```python
from build123d import *

# Parameters (mm, degrees)
CHAMFER_1_SIZE = 0.2
CHAMFER_2_SIZE = 0.1


with BuildPart() as part:
    # Эскиз1 → Повернуть1 (revolve)
    with BuildSketch(Plane.XY, mode=Mode.PRIVATE) as revolve_1_sk:
        Polygon((0, 0), (26, 0), (26, 2), (25, 2), (25, 1.7), (24.3, 1.7), (24.3, 2), (8, 2), (8, 3), (5.5, 3), (5.5, 2), (0, 2), align=None)
    revolve(revolve_1_sk.sketch.rotate(Axis((0, 0, 0), (1, 0, 0)), 90), axis=Axis((0, 0, 0), (1, 0, 0)))

    # Фаска1
    chamfer_1_edges = [part.edges().sort_by_distance(p)[0] for p in [
        (26, 0, -2),
        (0, 0, -2),
    ]]
    chamfer(chamfer_1_edges, length=CHAMFER_1_SIZE)

    # Фаска2
    chamfer_2_edges = [part.edges().sort_by_distance(p)[0] for p in [
        (24.3, 0, -2),
        (25, 0, -2),
    ]]
    chamfer(chamfer_2_edges, length=CHAMFER_2_SIZE)


solid = part.part
```
Geometry: final body of the model. Coordinates: model frame, mm. A direction names the side the tool comes from. Round coordinates to 2 decimals unless told otherwise and drop trailing zeros. Order: outer loops, then holes, each group sorted by start corner. A loop starts at its lowest first (then second) coordinate and runs counter-clockwise, first axis right, second up. Notation, with made-up numbers: (24, 8.5) -> (32, 8.5) arc R28 ccw to (32, 40.5) -> close; hole circle Ø8 at (30.5, 70.25). An arc over 180 degrees is marked (long way). Use one line per item in the form item = value. Start each with the question number.
1. Reachability of faces 4 (the face through (8, 2, -1)), 5 (the face through (3, 2, 0)), 6 (the face through (26, 0, 0)) from +Z, -Z, +X, -X, +Y, -Y: full face, straight path, thin tool, end or side. Return the list, or none.
2. Cut plane C-C (x = 21.5). Return the cut outline in (y, z), then the cut area to 3 significant figures.
3. Draft query along X for faces 1 (the face through (24.65, 1.66, -0.37)), 2 (the face through (5.5, 2, 1)), 3 (the face through (16, 2, 0)). Return one class per face: pulls with the +X half, pulls with the -X half, needs draft (parallel to the pull), parting line crosses it, or undercut.
4. Cut plane A-A (z = 0). Return the cut outline in (x, y), then the cut area to 3 significant figures.
5. Pin query (flat end, axial travel): pin 1 Ø1 at (x, z) = (22, -1) entering from -Y; pin 2 Ø1.5 at (x, y) = (15, 2) entering from -Z; pin 3 Ø1.1 at (y, z) = (0.5, 0) entering from -X. Return the tip coordinate at first contact, or that it passes through.
6. Line query: probe 1 along Y at (x, z) = (5, 0.15); probe 2 along X at (y, z) = (1.35, 2); probe 3 along Z at (x, y) = (12.5, 0.1). Output: solid intervals per line, ascending.
Solution:
q1.face_4 = +X
q1.face_5 = -X
q1.face_6 = +Z, -Z, +X, +Y, -Y
q2.outline = circle Ø4 at (0, 0)
q2.area = 12.6 mm^2
q3.face_1 = undercut
q3.face_2 = pulls with the -X half
q3.face_3 = needs draft
q4.outline = (0, -1.8) -> (0.2, -2) -> (5.5, -2) -> (5.5, -3) -> (8, -3) -> (8, -2) -> (24.2, -2) -> (24.3, -1.9) -> (24.3, -1.7) -> (25, -1.7) -> (25, -1.9) -> (25.1, -2) -> (25.8, -2) -> (26, -1.8) -> (26, 1.8) -> (25.8, 2) -> (25.1, 2) -> (25, 1.9) -> (25, 1.7) -> (24.3, 1.7) -> (24.3, 1.9) -> (24.2, 2) -> (8, 2) -> (8, 3) -> (5.5, 3) -> (5.5, 2) -> (0.2, 2) -> (0, 1.8) -> close
q4.area = 108 mm^2
q5.pin_1 = -1.94
q5.pin_2 = -1.56
q5.pin_3 = 0
q6.probe_1 = -1.99 to 1.99
q6.probe_2 = 5.5 to 8
q6.probe_3 = -2 to 2
